Check sheet for the modelled part. Datum: model origin and axes. Units: mm. Face numbers are marked on the shaded views. A direction names the side the tool comes from. Round coordinates to 2 decimals unless told otherwise and drop trailing zeros. Order: outer loops, then holes, each group sorted by start corner. A loop starts at its lowest first (then second) coordinate and runs counter-clockwise, first axis right, second up. Notation, with made-up numbers: M 88.5,35 L 130.5,35 A32 cw 130.5,74 Z; hole C 38.25,62 d5. An arc over 180 degrees is marked long. One line per item, written item: value. Start each with the question number.
(1) Thickness scan on L1, parallel to Y at x = 15, z = 13; L2, parallel to Z at x = 11.25, y = -19.5; L3, parallel to Z at x = 7, y = -20. Record the ranges inside material, lowest first.
(2) Cross-section at D-D, the plane y = -25.5. Enter the section's corners in (x, z) (3 decimals).
(3) Cross-section at B-B, the plane y = -20.5. Enter the section's corners in (x, z) (3 decimals).
(4) Cross-section at C-C, the plane z = 8. Enter the section's corners in (x, y).
(5) Access from +Z, -Z, +X, -X, +Y, -Y to the whole of each face (thin tool, end or side, straight path). Record for the marked faces 5 and 6.
(6) Release check for a two-part mould opening along X. For the marked faces 1, 2, 3 and 4 record: released by +X, released by -X, zero draft, split by the parting line, or undercut.
(7) Cross-section at A-A, the plane z = 16.25. Enter the section's corners in (x, y).
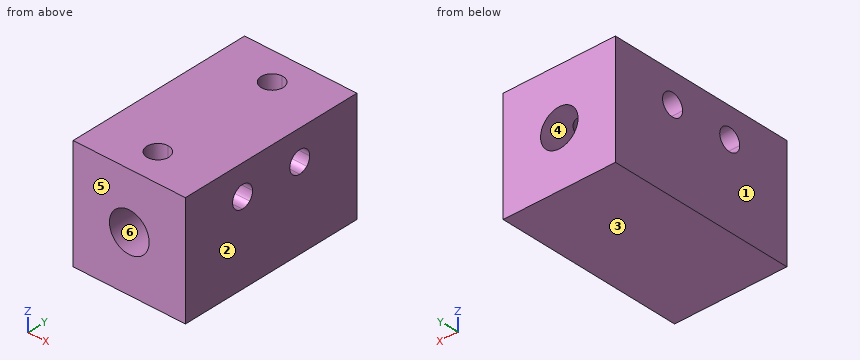
from build123d import *

# Parameters (mm, degrees)
F0_W     = 17.9605122421
F0_H     = 17.9605122421
F1_DEPTH = 30
F2_R     = 3.175
F3_DEPTH = 15
F4_R     = 3
F5_DEPTH = 15
F7_DEPTH = 10.5811646208
F9_DEPTH = 51.3227693737


with BuildPart() as f1:
    # F0 (on Front) → F1 (new body)
    with BuildSketch(Plane.XZ):
        with Locations((8.9802561211, 8.9802561211)):
            Rectangle(F0_W, F0_H)
    extrude(amount=F1_DEPTH)

    # F2 (on face) → F3 (cut)
    with BuildSketch(Plane.XZ.offset(30)):
        with Locations((8.9802561211, 8.9802561211)):
            Circle(F2_R)
    extrude(amount=-F3_DEPTH, mode=Mode.SUBTRACT)

    # F4 (on face) → F5 (cut)
    with BuildSketch(Plane(origin=(0, 0, 0), x_dir=(-1, 0, 0), z_dir=(0, 1, 0))):
        with Locations((-8.9802561211, 8.9802561211)):
            Circle(F4_R)
    extrude(amount=-F5_DEPTH, mode=Mode.SUBTRACT)

    # F6 (on face) → F7 (cut)
    with BuildSketch(Plane.XY.offset(17.9605122421)):
        with BuildLine():
            ThreePointArc((8.9802561211, -23.25), (7.2302561211, -25), (8.9802561211, -26.75))
            Line((8.9802561211, -26.75), (8.9802561211, -23.25))
        make_face()
        with BuildLine():
            Line((8.9802561211, -23.25), (8.9802561211, -26.75))
            ThreePointArc((8.9802561211, -26.75), (10.2176929881, -26.2374368671), (10.7302561211, -25))
            ThreePointArc((10.7302561211, -25), (10.2176929881, -23.7625631329), (8.9802561211, -23.25))
        make_face()
        with BuildLine():
            ThreePointArc((8.9802561211, -3.25), (7.2302561211, -5), (8.9802561211, -6.75))
            Line((8.9802561211, -6.75), (8.9802561211, -3.25))
        make_face()
        with BuildLine():
            Line((8.9802561211, -3.25), (8.9802561211, -6.75))
            ThreePointArc((8.9802561211, -6.75), (10.2176929881, -6.2374368671), (10.7302561211, -5))
            ThreePointArc((10.7302561211, -5), (10.2176929881, -3.7625631329), (8.9802561211, -3.25))
        make_face()
    extrude(amount=-F7_DEPTH, mode=Mode.SUBTRACT)

    # F8 (on face) → F9 (cut)
    with BuildSketch(Plane.YZ.offset(17.9605122421)):
        with BuildLine():
            ThreePointArc((-21.2362894379, 11.9046728878), (-20, 12.1552561211), (-18.7637105621, 11.9046728878))
            ThreePointArc((-18.7637105621, 11.9046728878), (-18.38352134, 12.4728109393), (-18.25, 13.1432561211))
            Line((-18.25, 13.1432561211), (-21.75, 13.1432561211))
            ThreePointArc((-21.75, 13.1432561211), (-21.61647866, 12.4728109393), (-21.2362894379, 11.9046728878))
        make_face()
        with BuildLine():
            ThreePointArc((-20, 11.3932561211), (-19.3310533124, 11.5261567645), (-18.7637105621, 11.9046728878))
            ThreePointArc((-18.7637105621, 11.9046728878), (-20, 12.1552561211), (-21.2362894379, 11.9046728878))
            ThreePointArc((-21.2362894379, 11.9046728878), (-20.6689466876, 11.5261567645), (-20, 11.3932561211))
        make_face()
        with BuildLine():
            Line((-21.75, 13.1432561211), (-18.25, 13.1432561211))
            ThreePointArc((-18.25, 13.1432561211), (-20, 14.8932561211), (-21.75, 13.1432561211))
        make_face()
        with BuildLine():
            ThreePointArc((-10.0000000112, 11.3932561211), (-9.3310533175, 11.5261567623), (-8.7637105621, 11.9046728878))
            ThreePointArc((-8.7637105621, 11.9046728878), (-10, 12.1552561211), (-11.2362894379, 11.9046728878))
            ThreePointArc((-11.2362894379, 11.9046728878), (-10.6689466928, 11.5261567666), (-10.0000000112, 11.3932561211))
        make_face()
        with BuildLine():
            ThreePointArc((-11.2362894379, 11.9046728878), (-10, 12.1552561211), (-8.7637105621, 11.9046728878))
            ThreePointArc((-8.7637105621, 11.9046728878), (-8.38352134, 12.4728109393), (-8.25, 13.1432561211))
            Line((-8.25, 13.1432561211), (-11.75, 13.1432561211))
            ThreePointArc((-11.75, 13.1432561211), (-11.61647866, 12.4728109393), (-11.2362894379, 11.9046728878))
        make_face()
        with BuildLine():
            Line((-11.75, 13.1432561211), (-8.25, 13.1432561211))
            ThreePointArc((-8.25, 13.1432561211), (-10, 14.8932561211), (-11.75, 13.1432561211))
        make_face()
    extrude(amount=-F9_DEPTH, mode=Mode.SUBTRACT)


solid = f1.part
Values found:
1. L1: -30 to -21.74, -18.26 to -11.74, -8.26 to 0
1. L2: 0 to 6.76, 11.2 to 11.47, 14.82 to 17.96
1. L3: 0 to 6.5, 14.89 to 17.96
2. outline: M 0,0 L 17.961,0 L 17.961,17.961 L 10.657,17.961 L 10.657,11.676 A3.175 cw long 7.303,11.676 L 7.303,17.961 L 0,17.961 Z
3. outline: M 0,0 L 17.961,0 L 17.961,11.466 L 10.955,11.466 A3.175 cw long 7.005,11.466 L 0,11.466 Z; M 0,14.82 L 17.961,14.82 L 17.961,17.961 L 0,17.961 Z
4. outline: M 0,-30 L 5.96,-30 L 5.96,-15 L 6.14,-15 L 6.14,0 L 0,0 Z; M 11.82,-15 L 12,-15 L 12,-30 L 17.96,-30 L 17.96,0 L 11.82,0 Z
5. face 5: +Z, -Z, +X, -X, -Y
5. face 6: -Y
6. face 1: released by -X
6. face 2: released by +X
6. face 3: zero draft
6. face 4: undercut
7. outline: M 0,-30 L 17.96,-30 L 17.96,0 L 0,0 Z; hole C 8.98,-25 d3.5; hole C 8.98,-5 d3.5
